Geometry check sheet. Reference: the model listing, model coordinates, mm. Give positions to 0.01 mm unless a question says otherwise; leave off trailing zeros. Write each loop counter-clockwise with the first axis right and the second up, starting at its lowest first coordinate (ties: lowest second). Pieces come first, ordered by that corner, then holes. Notation, with made-up numbers: M -5,51.5 L 43,51.5 A16 ccw 43,70.5 Z; hole C 1.25,60 d4. An arc over 180 degrees is marked long. One line per item, written item: value. Start each with the question number.
1. Scan lines: line 1 (Y direction, x = 21.5, z = 4.35); line 2 (Y direction, x = 15.5, z = 2.85); line 3 (X direction, y = 6.5, z = 1.4). Record each from-to range of solid material in increasing order.
2. Release check for a two-part mould opening along X. For faces 1 (the face through (-4.25, -17.8, 2.46)), 2 (the face through (23.846, 7.509, 2.274)), 3 (the face through (11.56, 14.19, 2.46)) record: pulls with the +X half, pulls with the -X half, needs draft (parallel to the pull), parting line crosses it, or undercut.
3. Gauge pin test, flat ends, axial feed: pin 1 (2.5 mm diameter, centred on y = 1.5, z = 3, fed in from -X); pin 2 (5.5 mm diameter, centred on x = -21, y = 1.5, fed in from +Z); pin 3 (1.9 mm diameter, centred on x = -5, y = -20, fed in from +Z); pin 4 (3 mm diameter, centred on x = 12.5, y = 7.5, fed in from +Z). Record the tip position at first contact, or that the pin passes through.
4. Cross-section at B-B on z = 1.85. Count the separate pieces of the cut face and the enclosed holes in it, then the cut area to 3 significant figures.
5. Cross-section at C-C on y = 0. Record the cut outline in (x, z).
6. Cross-section at A-A on x = 0. Record the cut outline in (y, z).
from build123d import *

# Parameters (mm, degrees)
F0_R     = 25
F0_W     = 5.2
F0_H     = 5.2
F0_R_2   = 15
F1_DEPTH = 5
F2_DEPTH = 0.5
F3_SIZE2 = 2.99999
F3_SIZE  = 4.99999


# Not quite as in the source:
# - a fillet or chamfer that OpenCascade refuses, or shapes differently, is made with other operations: its cross-section is extruded or revolved along the edge and cut away or added
# - a fillet or chamfer is up to 0.001 mm smaller than in the source, because OpenCascade refuses the exact size


with BuildPart() as f1:
    # F0 (on Top) → F1 (new body)
    with BuildSketch(Plane.XY):
        Circle(F0_R)
        Polygon((-12.7365232116, -19.9005898526), (-16.8020469205, -16.6584428829), (-13.5598999508, -12.5929191741), (-9.494376242, -15.8350661437), align=None, mode=Mode.SUBTRACT)
        Polygon((-2.8406685631, -23.4559822245), (-7.9102937065, -22.2988733679), (-6.7531848499, -17.2292482245), (-1.6835597066, -18.3863570811), align=None, mode=Mode.SUBTRACT)
        Polygon((-20.1097532349, -12.4036415956), (-22.3659486783, -7.7186034825), (-17.6809105652, -5.4624080391), (-15.4247151218, -10.1474461522), align=None, mode=Mode.SUBTRACT)
        Polygon((7.6178153328, -22.3656296481), (2.5481901895, -23.5227385047), (1.3910813329, -18.4531133613), (6.4607064762, -17.2960045047), align=None, mode=Mode.SUBTRACT)
        Polygon((16.5674974757, -16.8454898234), (12.5019737669, -20.0876367931), (9.2598267972, -16.0221130843), (13.3253505061, -12.7799661146), align=None, mode=Mode.SUBTRACT)
        Polygon((22.2357835565, -7.9888941429), (19.9795881131, -12.673932256), (15.29455, -10.4177368126), (17.5507454435, -5.7326986995), align=None, mode=Mode.SUBTRACT)
        with Locations((20.9, -0.15)):
            Rectangle(F0_W, F0_H, mode=Mode.SUBTRACT)
        with Locations((-20.9, 0.15)):
            Rectangle(F0_W, F0_H, mode=Mode.SUBTRACT)
        Polygon((-22.2357835565, 7.9888941429), (-19.9795881131, 12.673932256), (-15.29455, 10.4177368126), (-17.5507454435, 5.7326986995), align=None, mode=Mode.SUBTRACT)
        Polygon((-16.5674974757, 16.8454898234), (-12.5019737669, 20.0876367931), (-9.2598267972, 16.0221130843), (-13.3253505061, 12.7799661146), align=None, mode=Mode.SUBTRACT)
        Polygon((-7.6178153328, 22.3656296481), (-2.5481901895, 23.5227385047), (-1.3910813329, 18.4531133613), (-6.4607064762, 17.2960045047), align=None, mode=Mode.SUBTRACT)
        Circle(F0_R_2, mode=Mode.SUBTRACT)
        Polygon((20.1097532349, 12.4036415956), (22.3659486783, 7.7186034825), (17.6809105652, 5.4624080391), (15.4247151218, 10.1474461522), align=None, mode=Mode.SUBTRACT)
        Polygon((2.8406685631, 23.4559822245), (7.9102937065, 22.2988733679), (6.7531848499, 17.2292482245), (1.6835597066, 18.3863570811), align=None, mode=Mode.SUBTRACT)
        Polygon((12.7365232116, 19.9005898526), (16.8020469205, 16.6584428829), (13.5598999508, 12.5929191741), (9.494376242, 15.8350661437), align=None, mode=Mode.SUBTRACT)
    extrude(amount=F1_DEPTH)

    # F0 (on Top) → F2 (join)
    with BuildSketch(Plane.XY):
        Circle(F0_R)
        Polygon((-12.7365232116, -19.9005898526), (-16.8020469205, -16.6584428829), (-13.5598999508, -12.5929191741), (-9.494376242, -15.8350661437), align=None, mode=Mode.SUBTRACT)
        Polygon((-2.8406685631, -23.4559822245), (-7.9102937065, -22.2988733679), (-6.7531848499, -17.2292482245), (-1.6835597066, -18.3863570811), align=None, mode=Mode.SUBTRACT)
        Polygon((-20.1097532349, -12.4036415956), (-22.3659486783, -7.7186034825), (-17.6809105652, -5.4624080391), (-15.4247151218, -10.1474461522), align=None, mode=Mode.SUBTRACT)
        Polygon((7.6178153328, -22.3656296481), (2.5481901895, -23.5227385047), (1.3910813329, -18.4531133613), (6.4607064762, -17.2960045047), align=None, mode=Mode.SUBTRACT)
        Polygon((16.5674974757, -16.8454898234), (12.5019737669, -20.0876367931), (9.2598267972, -16.0221130843), (13.3253505061, -12.7799661146), align=None, mode=Mode.SUBTRACT)
        Polygon((22.2357835565, -7.9888941429), (19.9795881131, -12.673932256), (15.29455, -10.4177368126), (17.5507454435, -5.7326986995), align=None, mode=Mode.SUBTRACT)
        with Locations((20.9, -0.15)):
            Rectangle(F0_W, F0_H, mode=Mode.SUBTRACT)
        with Locations((-20.9, 0.15)):
            Rectangle(F0_W, F0_H, mode=Mode.SUBTRACT)
        Polygon((-22.2357835565, 7.9888941429), (-19.9795881131, 12.673932256), (-15.29455, 10.4177368126), (-17.5507454435, 5.7326986995), align=None, mode=Mode.SUBTRACT)
        Polygon((-16.5674974757, 16.8454898234), (-12.5019737669, 20.0876367931), (-9.2598267972, 16.0221130843), (-13.3253505061, 12.7799661146), align=None, mode=Mode.SUBTRACT)
        Polygon((-7.6178153328, 22.3656296481), (-2.5481901895, 23.5227385047), (-1.3910813329, 18.4531133613), (-6.4607064762, 17.2960045047), align=None, mode=Mode.SUBTRACT)
        Circle(F0_R_2, mode=Mode.SUBTRACT)
        Polygon((20.1097532349, 12.4036415956), (22.3659486783, 7.7186034825), (17.6809105652, 5.4624080391), (15.4247151218, 10.1474461522), align=None, mode=Mode.SUBTRACT)
        Polygon((2.8406685631, 23.4559822245), (7.9102937065, 22.2988733679), (6.7531848499, 17.2292482245), (1.6835597066, 18.3863570811), align=None, mode=Mode.SUBTRACT)
        Polygon((12.7365232116, 19.9005898526), (16.8020469205, 16.6584428829), (13.5598999508, 12.5929191741), (9.494376242, 15.8350661437), align=None, mode=Mode.SUBTRACT)
        Polygon((-15.29455, 10.4177368126), (-19.9795881131, 12.673932256), (-22.2357835565, 7.9888941429), (-17.5507454435, 5.7326986995), align=None)
        Polygon((-9.2598267972, 16.0221130843), (-12.5019737669, 20.0876367931), (-16.5674974757, 16.8454898234), (-13.3253505061, 12.7799661146), align=None)
        Polygon((-1.3910813329, 18.4531133613), (-2.5481901895, 23.5227385047), (-7.6178153328, 22.3656296481), (-6.4607064762, 17.2960045047), align=None)
        Polygon((6.7531848499, 17.2292482245), (7.9102937065, 22.2988733679), (2.8406685631, 23.4559822245), (1.6835597066, 18.3863570811), align=None)
        Polygon((13.5598999508, 12.5929191741), (16.8020469205, 16.6584428829), (12.7365232116, 19.9005898526), (9.494376242, 15.8350661437), align=None)
        Polygon((17.6809105652, 5.4624080391), (22.3659486783, 7.7186034825), (20.1097532349, 12.4036415956), (15.4247151218, 10.1474461522), align=None)
        with Locations((20.9, -0.15)):
            Rectangle(F0_W, F0_H)
        Polygon((15.29455, -10.4177368126), (19.9795881131, -12.673932256), (22.2357835565, -7.9888941429), (17.5507454435, -5.7326986995), align=None)
        Polygon((9.2598267972, -16.0221130843), (12.5019737669, -20.0876367931), (16.5674974757, -16.8454898234), (13.3253505061, -12.7799661146), align=None)
        with Locations((-20.9, 0.15)):
            Rectangle(F0_W, F0_H)
        Polygon((-13.5598999508, -12.5929191741), (-16.8020469205, -16.6584428829), (-12.7365232116, -19.9005898526), (-9.494376242, -15.8350661437), align=None)
        Polygon((-17.6809105652, -5.4624080391), (-22.3659486783, -7.7186034825), (-20.1097532349, -12.4036415956), (-15.4247151218, -10.1474461522), align=None)
        Polygon((-6.7531848499, -17.2292482245), (-7.9102937065, -22.2988733679), (-2.8406685631, -23.4559822245), (-1.6835597066, -18.3863570811), align=None)
        Polygon((1.3910813329, -18.4531133613), (2.5481901895, -23.5227385047), (7.6178153328, -22.3656296481), (6.4607064762, -17.2960045047), align=None)
    extrude(amount=-F2_DEPTH)

    # F3 (size 5 and 3 in the source; OpenCascade refuses exactly that, so slightly less here)
    f3_edges = [f1.edges().sort_by_distance(p)[0] for p in [
        (-15, 0, 5),
    ]]
    f3_side = f1.faces().sort_by_distance((-15, 0, 2.5))[0]
    chamfer(f3_edges, length=F3_SIZE, length2=F3_SIZE2, reference=f3_side)

    # F4: chamfer of 1 on 3 edges, made by hand

    # F4_s1 → F4_t2 (revolve, cut)
    with BuildSketch(Plane.XZ):
        Polygon((24, 5), (25, 4), (25, 5), align=None)
    revolve(axis=Axis((0, 0, 5), (0, 0, 1)), mode=Mode.SUBTRACT)

    # F4_s3 → F4_t4 (revolve, cut)
    with BuildSketch(Plane.XZ):
        Polygon((25, 0.5), (24, -0.5), (25, -0.5), align=None)
    revolve(axis=Axis((0, 0, -0.5), (0, 0, 1)), mode=Mode.SUBTRACT)

    # F4_s5 → F4_t6 (revolve, cut)
    with BuildSketch(Plane.XZ):
        Polygon((15, 0.5), (16, -0.5), (15, -0.5), align=None)
    revolve(axis=Axis((0, 0, -0.5), (0, 0, 1)), mode=Mode.SUBTRACT)


solid = f1.part
Report:
1. line 1: y = -12.06 to -9.52, -7.63 to -2.75, 2.45 to 7.3, 9.52 to 12.06
1. line 2: y = -19.62 to -17.7, -15.51 to -10.52, -9.99 to -6.24, 6.24 to 9.99, 10.18 to 15.03, 17.7 to 19.62
1. line 3: x = -24.14 to -19.14, -17.18 to -14.44, 14.44 to 17.18, 19.84 to 24.14
2. face 1: undercut
2. face 2: parting line crosses it
2. face 3: undercut
3. pin 1: stops at x = -25
3. pin 2: stops at z = 5
3. pin 3: stops at z = 0
3. pin 4: stops at z = 1.8
4. separate pieces: 1
4. enclosed holes: 15
4. area: 770 mm^2
5. outline: M -25,0.5 L -24,-0.5 L -16,-0.5 L -15.19,0.31 L -18,5 L -18.3,5 L -18.3,0 L -23.5,0 L -23.5,5 L -24,5 L -25,4 Z; M 15.19,0.31 L 16,-0.5 L 24,-0.5 L 25,0.5 L 25,4 L 24,5 L 23.5,5 L 23.5,0 L 18.3,0 L 18.3,5 L 18,5 Z
6. outline: M -25,0.5 L -24,-0.5 L -16,-0.5 L -15.19,0.31 L -18,5 L -24,5 L -25,4 Z; M 15.19,0.31 L 16,-0.5 L 24,-0.5 L 25,0.5 L 25,4 L 24,5 L 18,5 Z
